Geometry: final body of the model. Coordinates: model frame, mm. A direction names the side the tool comes from. Coordinates: 2 decimals unless noted, no trailing zeros. Write each loop counter-clockwise with the first axis right and the second up, starting at its lowest first coordinate (ties: lowest second). Pieces come first, ordered by that corner, then holes.
from build123d import *

# Parameters (mm, degrees)
F0_R      = 10
F0_W      = 21.869414486
F0_H      = 18.1213598698
F1_DEPTH  = 17
F3_DEPTH  = 15
F4_W      = 7
F4_H      = 3
F5_DEPTH  = 5
F7_DEPTH  = 14
F8_SIZE   = 2
F9_W      = 18
F9_H      = 6
F10_DEPTH = 6


# Not quite as in the source:
# - a feature names something its author has since deleted; it is built from what else it names


with BuildPart() as f1:
    # F0 (on Top) → F1 (new body)
    with BuildSketch(Plane.XY):
        Polygon((27, -38.3339710534), (27, 50.5), (-27, 50.5), (-27, -50.5), (27, -50.5), align=None)
        Polygon((25, -29.2732911184), (25, -38.3339710534), (25, -47.3946509883), (3.130585514, -47.3946509883), (3.130585514, -29.2732911184), align=None, mode=Mode.SUBTRACT)
        Circle(F0_R, mode=Mode.SUBTRACT)
        with BuildLine():
            ThreePointArc((17.75, 0), (16, -1.75), (14.25, 0))
            ThreePointArc((14.25, 0), (16, 1.75), (17.75, 0))
        make_face(mode=Mode.SUBTRACT)
        with Locations((14.065292757, 38.3339710534)):
            Rectangle(F0_W, F0_H, mode=Mode.SUBTRACT)
    extrude(amount=F1_DEPTH)

    # F2 (on face) → F3 (cut)
    with BuildSketch(Plane(origin=(0, 0, 0), x_dir=(1, 0, 0), z_dir=(0, 0, -1))):
        Polygon((7.125, 26), (7.125, 0), (7.125, -26), (24.875, -26), (24.875, 23), (17.875, 23), (17.875, 26), align=None)
        with BuildLine():
            ThreePointArc((20.5, 0), (16, -4.5), (11.5, 0))
            ThreePointArc((11.5, 0), (16, 4.5), (20.5, 0))
        make_face(mode=Mode.SUBTRACT)
        with BuildLine():
            Line((-11.8641304348, -45), (-11.8641304348, 0))
            Line((-11.8641304348, 0), (-11.8641304348, 45))
            Line((-11.8641304348, 45), (-14.3641304348, 45))
            Line((-14.3641304348, 45), (-14.3641304348, 46))
            Line((-14.3641304348, 46), (-11.8431356333, 46))
            Line((-11.8431356333, 46), (-11.8431356333, 47))
            Line((-11.8431356333, 47), (-14.3641304348, 47))
            ThreePointArc((-14.3641304348, 47), (-17, 49.6358695652), (-19.6358695652, 47))
            Line((-19.6358695652, 47), (-22.1358695652, 47))
            Line((-22.1358695652, 47), (-22.1358695652, 46))
            Line((-22.1358695652, 46), (-19.6358695652, 46))
            Line((-19.6358695652, 46), (-19.6358695652, 45))
            Line((-19.6358695652, 45), (-22.1358695652, 45))
            Line((-22.1358695652, 45), (-22.1358695652, -45))
            Line((-22.1358695652, -45), (-19.6358695652, -45))
            Line((-19.6358695652, -45), (-19.6358695652, -46))
            Line((-19.6358695652, -46), (-22.1358695652, -46))
            Line((-22.1358695652, -46), (-22.1358695652, -47))
            Line((-22.1358695652, -47), (-19.6358695652, -47))
            ThreePointArc((-19.6358695652, -47), (-17, -49.6358695652), (-14.3641304348, -47))
            Line((-14.3641304348, -47), (-11.8431356333, -47))
            Line((-11.8431356333, -47), (-11.8431356333, -46))
            Line((-11.8431356333, -46), (-14.3641304348, -46))
            Line((-14.3641304348, -46), (-14.3641304348, -45))
            Line((-14.3641304348, -45), (-11.8641304348, -45))
        make_face()
    extrude(amount=-F3_DEPTH, mode=Mode.SUBTRACT)

    # F4 (on face) → F5 (cut)
    with BuildSketch(Plane(origin=(0, 0, 0), x_dir=(1, 0, 0), z_dir=(0, 0, -1))):
        with Locations((21.5, 24.5)):
            Rectangle(F4_W, F4_H)
        with BuildLine():
            Line((0, 29.1349645704), (0, 39.6236035006))
            ThreePointArc((0, 39.6236035006), (-2.9289321881, 46.6946713125), (-10, 49.6236035006))
            Line((-10, 49.6236035006), (-17, 49.6358695652))
            Line((-17, 49.6358695652), (-17, 47.6358695652))
            Line((-17, 47.6358695652), (-10, 47.6358695652))
            ThreePointArc((-10, 47.6358695652), (-4.3388107028, 45.2883854424), (-2.0000094035, 39.6236035006))
            Line((-2.0000094035, 39.6236035006), (-2.0000094035, 29.1349645704))
            ThreePointArc((-2.0000094035, 29.1349645704), (0.5848933582, 22.5223852264), (7.1590254083, 19.8412071913))
            Line((7.1590254083, 19.8412071913), (7.125, 21.6599348028))
            ThreePointArc((7.125, 21.6599348028), (1.9168065811, 23.8288183935), (0, 29.1349645704))
        make_face()
        with BuildLine():
            ThreePointArc((7.1590254083, -19.8412071913), (0.5848933582, -22.5223852264), (-2.0000094035, -29.1349645704))
            Line((-2.0000094035, -29.1349645704), (-2.0000094035, -39.6236035006))
            ThreePointArc((-2.0000094035, -39.6236035006), (-4.3388107028, -45.2883854424), (-10, -47.6358695652))
            Line((-10, -47.6358695652), (-17, -47.6358695652))
            Line((-17, -47.6358695652), (-17, -49.6358695652))
            Line((-17, -49.6358695652), (-10, -49.6236035006))
            ThreePointArc((-10, -49.6236035006), (-2.9289321881, -46.6946713125), (0, -39.6236035006))
            Line((0, -39.6236035006), (0, -29.1349645704))
            ThreePointArc((0, -29.1349645704), (1.9168065811, -23.8288183935), (7.125, -21.6599348028))
            Line((7.125, -21.6599348028), (7.1590254083, -19.8412071913))
        make_face()
    extrude(amount=-F5_DEPTH, mode=Mode.SUBTRACT)

    # F6 (on face) → F7 (cut)
    with BuildSketch(Plane(origin=(0, 0, 0), x_dir=(1, 0, 0), z_dir=(0, 0, -1))):
        with BuildLine():
            ThreePointArc((24.25, 24.75), (23.5, 25.5), (22.75, 24.75))
            ThreePointArc((22.75, 24.75), (23.5, 24), (24.25, 24.75))
        make_face()
        Polygon((7.125, -26), (7.125, -36.75), (7.125, -47.5), (24.875, -47.5), (24.875, -26), align=None)
    extrude(amount=-F7_DEPTH, mode=Mode.SUBTRACT)

    # F8
    f8_edges = [f1.edges().sort_by_distance(p)[0] for p in [
        (14.25, 0, 0),
    ]]
    chamfer(f8_edges, length=F8_SIZE)

    # F9 (on face) → F10 (join)
    with BuildSketch(Plane.XY.offset(17)):
        with Locations((16.0392038773, 22.9714149609)):
            Rectangle(F9_W, F9_H)
    extrude(amount=-F10_DEPTH)


solid = f1.part
Item 1: Pull-direction query (Y, two-part tool) for faces 4 (the flat face through (-21, -46, 7)), 5 (the flat face through (0, 50.5, 8)), 6 (the flat face through (-12, 47.636, 2)), 7 (the flat face through (-11, 1, 0)); classes: released by +Y, released by -Y, zero draft, split by the parting line, or undercut.
Derived:
face 4: undercut
face 5: released by +Y
face 6: undercut
face 7: zero draft
Item 2: Set-up query: faces 1 (the flat face through (15, 4, 0)), 2 (the flat face through (17.875, -24, 7)), 3 (the flat face through (3.131, -38, 8)). Return all of +Z, -Z, +X, -X, +Y, -Y with unobstructed straight access to the full face (end or side cutting, diameter ignored); none if empty.
Derived:
face 1: -Z, +X, -X, +Y, -Y
face 2: -Z
face 3: +Z, -Z
Item 3: Material intervals for probe 1 along Y at (x, z) = (23.5, 8.75); probe 2 along X at (y, z) = (-41.5, 8.25); probe 3 along Y at (x, z) = (16, 10.75), sorted ascending.
Derived:
probe 1: y = -50.5 to -47.39, -29.27 to -25.5, -24 to -23, 47.5 to 50.5
probe 2: x = -27 to -22.14, -11.86 to 3.13, 25 to 27
probe 3: y = -50.5 to -47.39, -29.27 to -26, -4.5 to -1.75, 1.75 to 4.5, 47.5 to 50.5
Item 4: Pin query (flat end, axial travel): pin 1 (5 mm diameter, centred on x = 9.5, y = 23, fed in from -Z); pin 2 (5 mm diameter, centred on x = 12, y = 23.5, fed in from -Z). Return the tip coordinate at first contact, or that it passes through.
Derived:
pin 1: stops at z = 0
pin 2: stops at z = 11
Item 5: Section A-A, the plane y = -35.5. Output: boundary loops of the cut face in (x, z), plus the area to 3 significant figures.
Derived:
outline: (-27, 0) - (-22.14, 0) - (-22.14, 15) - (-11.86, 15) - (-11.86, 0) - (-2, 0) - (-2, 5) - (0, 5) - (0, 0) - (3.13, 0) - (3.13, 17) - (-27, 17) - close; (25, 0) - (27, 0) - (27, 17) - (25, 17) - close
area: 382 mm2
Item 6: Section B-B, the plane x = 16. State how many separate pieces and enclosed holes the cut face has, plus the area to 3 significant figures.
Derived:
separate pieces: 4
enclosed holes: 0
area: 369 mm2
